from build123d import *

# Parameters (mm, degrees)
SKETCH8_R           = 2.5
SKETCH8_R_2         = 2.3
BOSS_EXTRUDE5_DEPTH = 3


with BuildPart() as part:
    # Sketch8 → Boss-Extrude5 (new body)
    # profile 1 of 7: a face of its own
    with BuildSketch(Plane(origin=(0, 0, 0), x_dir=(1, 0, 0), z_dir=(0, 1, 0))):
        with BuildLine():
            ThreePointArc((-4.330127019, 2.5), (-2.5, 4.330127019), (0, 5))
            Line((0, 5), (2.886751346, 5))
            Line((2.886751346, 5), (-53.669872981, 102.958946839))
            ThreePointArc((-53.669872981, 102.958946839), (-60.5, 104.789073858), (-62.330127019, 97.958946839))
            Line((-62.330127019, 97.958946839), (-5.773502692, 0))
            Line((-5.773502692, 0), (-4.330127019, 2.5))
        make_face()
        with Locations(Location((-58, 100.458946839, 0), (0, 0, 270))):
            Circle(SKETCH8_R, mode=Mode.SUBTRACT)
    # profile 2 of 7: a face of its own
    with BuildSketch(Plane(origin=(0, 0, 0), x_dir=(1, 0, 0), z_dir=(0, 1, 0))):
        with BuildLine():
            Line((116, 5), (2.886751346, 5))
            Line((2.886751346, 5), (4.330127019, 2.5))
            ThreePointArc((4.330127019, 2.5), (5, 0), (4.330127019, -2.5))
            Line((4.330127019, -2.5), (2.886751346, -5))
            Line((2.886751346, -5), (116, -5))
            ThreePointArc((116, -5), (121, 0), (116, 5))
        make_face()
        with Locations(Location((116, 0, 0), (0, 0, 270))):
            Circle(SKETCH8_R, mode=Mode.SUBTRACT)
    # profile 3 of 7: a face of its own
    with BuildSketch(Plane(origin=(0, 0, 0), x_dir=(1, 0, 0), z_dir=(0, 1, 0))):
        with BuildLine():
            Line((-4.330127019, -2.5), (-5.773502692, 0))
            Line((-5.773502692, 0), (-62.330127019, -97.958946839))
            ThreePointArc((-62.330127019, -97.958946839), (-60.5, -104.789073858), (-53.669872981, -102.958946839))
            Line((-53.669872981, -102.958946839), (2.886751346, -5))
            Line((2.886751346, -5), (0, -5))
            ThreePointArc((0, -5), (-2.5, -4.330127019), (-4.330127019, -2.5))
        make_face()
        with Locations(Location((-58, -100.458946839, 0), (0, 0, 270))):
            Circle(SKETCH8_R, mode=Mode.SUBTRACT)
    # profile 4 of 7: a face of its own
    with BuildSketch(Plane(origin=(0, 0, 0), x_dir=(1, 0, 0), z_dir=(0, 1, 0))):
        with BuildLine():
            ThreePointArc((4.330127019, 2.5), (2.5, 4.330127019), (0, 5))
            ThreePointArc((0, 5), (-2.5, 4.330127019), (-4.330127019, 2.5))
            ThreePointArc((-4.330127019, 2.5), (-5, 0), (-4.330127019, -2.5))
            ThreePointArc((-4.330127019, -2.5), (-2.5, -4.330127019), (0, -5))
            ThreePointArc((0, -5), (2.5, -4.330127019), (4.330127019, -2.5))
            ThreePointArc((4.330127019, -2.5), (5, 0), (4.330127019, 2.5))
        make_face()
        with Locations(Location((0, 0, 0), (0, 0, 270))):
            Circle(SKETCH8_R_2, mode=Mode.SUBTRACT)
    # profile 5 of 7: a face of its own
    with BuildSketch(Plane(origin=(0, 0, 0), x_dir=(1, 0, 0), z_dir=(0, 1, 0))):
        with BuildLine():
            Line((2.886751346, 5), (0, 5))
            ThreePointArc((0, 5), (2.5, 4.330127019), (4.330127019, 2.5))
            Line((4.330127019, 2.5), (2.886751346, 5))
        make_face()
    # profile 6 of 7: a face of its own
    with BuildSketch(Plane(origin=(0, 0, 0), x_dir=(1, 0, 0), z_dir=(0, 1, 0))):
        with BuildLine():
            ThreePointArc((-4.330127019, -2.5), (-5, 0), (-4.330127019, 2.5))
            Line((-4.330127019, 2.5), (-5.773502692, 0))
            Line((-5.773502692, 0), (-4.330127019, -2.5))
        make_face()
    # profile 7 of 7: a face of its own
    with BuildSketch(Plane(origin=(0, 0, 0), x_dir=(1, 0, 0), z_dir=(0, 1, 0))):
        with BuildLine():
            Line((2.886751346, -5), (4.330127019, -2.5))
            ThreePointArc((4.330127019, -2.5), (2.5, -4.330127019), (0, -5))
            Line((0, -5), (2.886751346, -5))
        make_face()
    extrude(amount=BOSS_EXTRUDE5_DEPTH)


solid = part.part
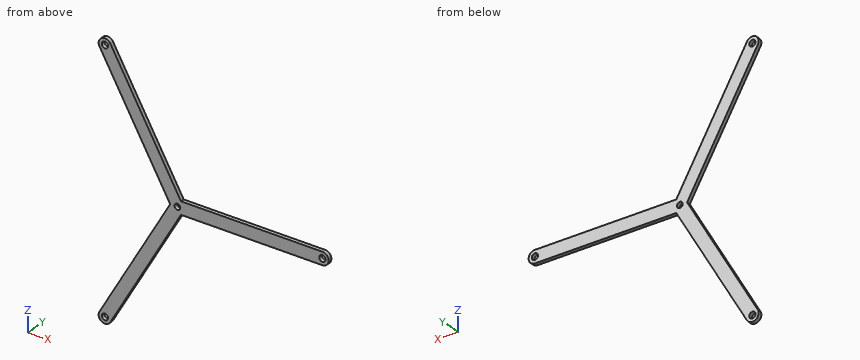
Can you work these out from the model? Positions are in its coordinate system, mm. Give positions to 0.01 mm unless a question says otherwise; leave off trailing zeros. Order: outer loops, then holes, each group sorted by start corner. A loop starts at its lowest first (then second) coordinate and runs counter-clockwise, first axis right, second up. Notation, with made-up numbers: M 87,87 L 118,87 A12 cw 118,106 Z; hole C 30.5,26.5 d6. An arc over 180 degrees is marked long. One line per item, written item: value.
Item 1: If we section it at B-B on x = -31.5: Write out the boundary of the cut face in (y, z).
Verdict:
outline: M 0,-64.56 L 3,-64.56 L 3,-44.56 L 0,-44.56 Z; M 0,44.56 L 3,44.56 L 3,64.56 L 0,64.56 Z
Item 2: Please list where these lines run through material, in increasing order: line 1 (X direction, y = 2.4, z = 0); line 2 (Z direction, x = 46, y = 2.45); line 3 (Z direction, x = -19.5, y = 2.3) (3 decimals).
Verdict:
line 1: -5.77 to -2.3, 2.3 to 113.5, 118.5 to 121
line 2: -5 to 5
line 3: -43.775 to -23.775, 23.775 to 43.775
Item 3: If we section it at D-D on x = 100: Write out the boundary of the cut face in (y, z), and give its area (3 significant figures).
Verdict:
outline: M 0,-5 L 3,-5 L 3,5 L 0,5 Z
area: 30.0 mm2
Item 4: If we section it at C-C on x = -58: Write out the boundary of the cut face in (y, z).
Verdict:
outline: M 0,-105.46 L 3,-105.46 L 3,-102.96 L 0,-102.96 Z; M 0,-97.96 L 3,-97.96 L 3,-90.46 L 0,-90.46 Z; M 0,90.46 L 3,90.46 L 3,97.96 L 0,97.96 Z; M 0,102.96 L 3,102.96 L 3,105.46 L 0,105.46 Z
Item 5: If we section it at A-A on y = 1.55: Write out the boundary of the cut face in (x, z), and give its area (3 significant figures).
Verdict:
outline: M -62.33,-97.96 A5 ccw -53.67,-102.96 L 2.89,-5 L 116,-5 A5 ccw 116,5 L 2.89,5 L -53.67,102.96 A5 ccw -62.33,97.96 L -5.77,0 Z; hole C -58,-100.46 d5; hole C -58,100.46 d5; hole C 0,0 d4.6; hole C 116,0 d5
area: 3,480 mm2
Item 6: For pin 1 (0.9 mm diameter, centred on x = 81, y = 1, fed in from +Z); pin 2 (1.5 mm diameter, centred on x = 38.5, y = 1, fed in from -Z), each with a flat end and sliding along its axis, tell me the tip position at first contact or that it passes through.
Verdict:
pin 1: z = 5
pin 2: z = -5
